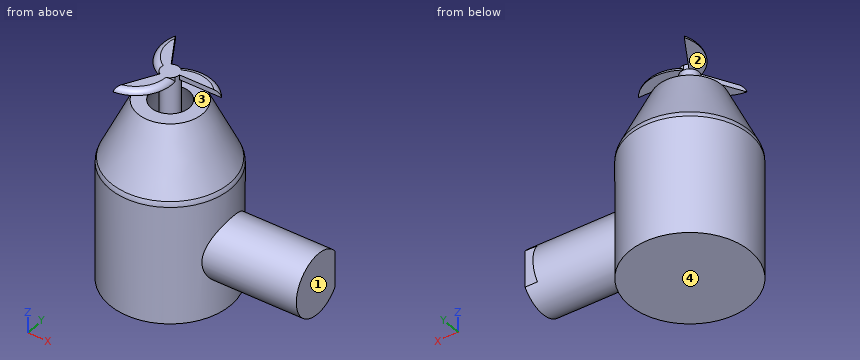
from build123d import *

# Parameters (mm, degrees)
SKETCH1_R                     = 50
BOSS_EXTRUDE1_DEPTH           = 100
BOSS_EXTRUDE1_OTHER_WAY_DEPTH = 50
BOSS_EXTRUDE1_OTHER_WAY_TAPER = 25
FILLET1_R                     = 10
SKETCH2_R                     = 7.5
BOSS_EXTRUDE2_DEPTH           = 160
SKETCH3_R                     = 7.5
BOSS_EXTRUDE3_DEPTH           = 4
FILLET2_R                     = 5
SKETCH4_R                     = 25
BOSS_EXTRUDE4_DEPTH           = 120
CUT_EXTRUDE2_START            = -10
CUT_EXTRUDE2_DEPTH            = 10


with BuildPart() as part:
    # Sketch1 → Boss-Extrude1 (new body)
    with BuildSketch(Plane.XY):
        Circle(SKETCH1_R)
    extrude(amount=-BOSS_EXTRUDE1_DEPTH)

    # Sketch1 → Boss-Extrude1 other way (add)
    with BuildSketch(Plane.XY):
        Circle(SKETCH1_R)
    extrude(amount=BOSS_EXTRUDE1_OTHER_WAY_DEPTH, taper=BOSS_EXTRUDE1_OTHER_WAY_TAPER)

    # Fillet1
    fillet1_edges = [part.edges().sort_by_distance(p)[0] for p in [
        (-50, 0, 0),
    ]]
    fillet(fillet1_edges, radius=FILLET1_R)

    # Shell2: read off the stored shape, not the designer's step
    # Shell2 outline → Shell2 (revolve, cut)
    with BuildSketch(Plane.XZ):
        Polygon((0, -90), (40, -90), (40, -2.216946626), (15.650837903, 50), (0, 50), align=None)
    revolve(axis=Axis((0, 0, 0), (0, 0, 1)), mode=Mode.SUBTRACT)

    # Sketch2 → Boss-Extrude2 (add)
    with BuildSketch(Plane.XY.offset(-90)):
        with Locations(Location((0, 0, 0), (0, 0, 180))):
            Circle(SKETCH2_R)
    extrude(amount=BOSS_EXTRUDE2_DEPTH)

    # Sketch3 → Boss-Extrude3 (add)
    with BuildSketch(Plane.XY.offset(70)):
        with BuildLine():
            ThreePointArc((0, 7.5), (5.303300859, 5.303300859), (7.5, 0))
            Line((7.5, 0), (41.895706174, 0))
            ThreePointArc((41.895706174, 0), (22.501153946, 12.426884851), (0, 7.5))
        make_face()
        with BuildLine():
            ThreePointArc((-6.495190528, -3.75), (-7.244443697, 1.941142838), (-3.75, 6.495190528))
            Line((-3.75, 6.495190528), (-20.947853087, 36.282745856))
            ThreePointArc((-20.947853087, 36.282745856), (-22.012574944, 13.273128506), (-6.495190528, -3.75))
        make_face()
        with BuildLine():
            ThreePointArc((-20.947853087, -36.282745856), (-0.488579002, -25.700013357), (6.495190528, -3.75))
            ThreePointArc((6.495190528, -3.75), (1.941142838, -7.244443697), (-3.75, -6.495190528))
            Line((-3.75, -6.495190528), (-20.947853087, -36.282745856))
        make_face()
        Circle(SKETCH3_R)
    extrude(amount=BOSS_EXTRUDE3_DEPTH)

    # Fillet2
    # the kernel refuses this fillet: 5 mm, written as the material it takes off along each edge
    with BuildSketch(Plane(origin=(17.197853087, -17.197853087, 74), x_dir=(0.979838516120554, 0.1997910967152214, 0), z_dir=(0.1997910967152214, -0.979838516120554, 0))) as fillet2_piece_1_section:
        with BuildLine():
            CenterArc((25.196702894, -5), FILLET2_R, 11.536959033, 78.463040967)
            Line((30.09568238, -4), (30.09568238, 0))
            Line((30.09568238, 0), (25.196702894, 0))
        make_face()
    fillet2_piece_1 = revolve(axis=Axis((17.197853087, -17.197853087, 74), (0, 0, 1)), revolution_arc=136.651808839, mode=Mode.PRIVATE)
    fillet2_piece_1 = fillet2_piece_1 - Plane(origin=(0, 0, 74), x_dir=(-1, 0, 0), z_dir=(0, 0, -1)) * Cylinder(7.5, 121, mode=Mode.PRIVATE)
    fillet2_piece_1 = split(fillet2_piece_1, bisect_by=Plane(origin=(17.197853087, 0, 74), z_dir=(0, 1, 0)), keep=Keep.TOP, mode=Mode.PRIVATE)
    add(fillet2_piece_1, mode=Mode.SUBTRACT)
    with BuildSketch(Plane(origin=(-23.492704207, -6.29485112, 74), x_dir=(-0.31689509285493905, -0.9484605949244596, 0), z_dir=(-0.9484605949244596, 0.31689509285493905, 0))) as fillet2_piece_2_section:
        with BuildLine():
            CenterArc((25.196702894, -5), FILLET2_R, 11.536959033, 78.463040967)
            Line((30.09568238, -4), (30.09568238, 0))
            Line((30.09568238, 0), (25.196702894, 0))
        make_face()
    fillet2_piece_2 = revolve(axis=Axis((-23.492704207, -6.29485112, 74), (0, 0, 1)), revolution_arc=136.651808839, mode=Mode.PRIVATE)
    fillet2_piece_2 = fillet2_piece_2 - Plane(origin=(0, 0, 74), x_dir=(-1, 0, 0), z_dir=(0, 0, -1)) * Cylinder(7.5, 121, mode=Mode.PRIVATE)
    fillet2_piece_2 = split(fillet2_piece_2, bisect_by=Plane(origin=(-8.598926543, -14.893777664, 74), z_dir=(0.8660254037844364, -0.500000000000004, 0)), keep=Keep.TOP, mode=Mode.PRIVATE)
    add(fillet2_piece_2, mode=Mode.SUBTRACT)
    with BuildSketch(Plane(origin=(6.29485112, 23.492704207, 74), x_dir=(-0.6629434232656098, 0.7486694982092396, 0), z_dir=(0.7486694982092396, 0.6629434232656098, 0))) as fillet2_piece_3_section:
        with BuildLine():
            CenterArc((25.196702894, -5), FILLET2_R, 11.536959033, 78.463040967)
            Line((25.196702894, 0), (30.09568238, 0))
            Line((30.09568238, 0), (30.09568238, -4))
        make_face()
    fillet2_piece_3 = revolve(axis=Axis((6.29485112, 23.492704207, 74), (0, 0, 1)), revolution_arc=136.651808839, mode=Mode.PRIVATE)
    fillet2_piece_3 = fillet2_piece_3 - Plane(origin=(0, 0, 74), x_dir=(-1, 0, 0), z_dir=(0, 0, -1)) * Cylinder(7.5, 121, mode=Mode.PRIVATE)
    fillet2_piece_3 = split(fillet2_piece_3, bisect_by=Plane(origin=(-8.598926543, 14.893777664, 74), z_dir=(-0.8660254037844434, -0.49999999999999206, 0)), keep=Keep.TOP, mode=Mode.PRIVATE)
    add(fillet2_piece_3, mode=Mode.SUBTRACT)

    # Sketch4 → Boss-Extrude4 (add)
    with BuildSketch(Plane(origin=(0, 0, 0), x_dir=(0, 0, -1), z_dir=(1, 0, 0))):
        with Locations(Location((51.895913136, 0, 0), (0, 0, 180))):
            Circle(SKETCH4_R)
    extrude(amount=BOSS_EXTRUDE4_DEPTH)

    # Sketch5 → Cut-Extrude2 (cut)
    with BuildSketch(Plane(origin=(120, 0, 0), x_dir=(0, 0, -1), z_dir=(1, 0, 0)).offset(CUT_EXTRUDE2_START)):
        with BuildLine():
            Line((36.699086206, 19.850855177), (67.092740066, 19.850855177))
            ThreePointArc((67.092740066, 19.850855177), (51.895913136, 25), (36.699086206, 19.850855177))
        make_face()
    extrude(amount=CUT_EXTRUDE2_DEPTH, mode=Mode.SUBTRACT)


solid = part.part
Part model, mm, in its own coordinate system. Face numbers are marked on the shaded views. Give positions to 0.01 mm unless a question says otherwise; leave off trailing zeros. Order: outer loops, then holes, each group sorted by start corner. A loop starts at its lowest first (then second) coordinate and runs counter-clockwise, first axis right, second up. Notation, with made-up numbers: (-38, -27) - (-14, -27) arc R26 cw to (-14, 3) - close; hole circle Ø3 at (-20, -29.75). An arc over 180 degrees is marked (long way). Use a Markdown table: item, result.
1) Saw through at D-D on z = 23.5. List the corners of the cut face in (x, y).
Checked values:
| item | result |
|---|---|
| outline | circle Ø78.08 at (0, 0); circle Ø15 at (0, 0); hole circle Ø56.02 at (0, 0) |
2) Two-plate mould, pull along Z, no slides. Class the marked faces 1, 2, 3 and 4: +Z half, -Z half, draft (parallel to the pull), parting line (faces both ways), or undercut.
Checked values:
| item | result |
|---|---|
| face 1 | draft |
| face 2 | undercut |
| face 3 | undercut |
| face 4 | -Z half |
3) Saw through at B-B on z = -53.5. List the corners of the cut face in (x, y), plus the area to 3 significant figures.
Checked values:
| item | result |
|---|---|
| outline | (43.33, -24.95) - (120, -24.95) - (120, 19.85) - (110, 19.85) - (110, 24.95) - (43.33, 24.95) arc R50 ccw (long way) to start; hole (0, -24.95) - (0, -7.5) arc R7.5 cw to (0, 7.5) - (0, 24.95) - (31.27, 24.95) arc R40 ccw (long way) to (31.27, -24.95) - close |
| area | 8,320 mm² |
4) Flat gauge pins, fed straight in: P1, Ø4, axis at x = 13, z = -41, coming from the -Y side (3 decimals); P2, Ø1, axis at x = 47, y = 14.5, coming from the +Z side; P3, Ø3, axis at x = 31, z = 72, coming from the -Y side. Where does each tip first touch, or does it go through?
Checked values:
| item | result |
|---|---|
| P1 | y = -48.775 |
| P2 | z = 2.82 |
| P3 | y = 0 |
5) Saw through at A-A on z = -10. List the corners of the cut face in (x, y).
Checked values:
| item | result |
|---|---|
| outline | circle Ø100 at (0, 0); circle Ø15 at (0, 0); hole circle Ø80 at (0, 0) |
6) Probe L1, parallel to Y at x = 0, z = -25; L2, parallel to Z at x = 12.5, y = 20.5 (3 decimals); L3, parallel to X at y = 17.5, z = 20.5. List the from-to ranges inside material, lowest first. Write a range as from..to.
Checked values:
| item | result |
|---|---|
| L1 | -50..-40, -7.5..7.5, 40..50 |
| L2 | -100..-90, -66.205..-37.587, 32.073..50 |
| L3 | -36.46..-23.63, 23.63..36.46 |
7) Saw through at C-C on x = 82.5. List the corners of the cut face in (y, z), plus the area to 3 significant figures.
Checked values:
| item | result |
|---|---|
| outline | circle Ø50 at (0, -51.9) |
| area | 1,960 mm² |
